Geometry check sheet. Reference: drawing and pictorial views, mm from the part's lowest x, y, z. A direction names the side the tool comes from. Round coordinates to 2 decimals unless told otherwise and drop trailing zeros. Write each loop counter-clockwise with the first axis right and the second up, starting at its lowest first coordinate (ties: lowest second). Pieces come first, ordered by that corner, then holes. Notation, with made-up numbers: M -37.5,89.5 L 1.5,89.5 A17 ccw 1.5,112.5 Z; hole C -39.75,5.25 d5. An arc over 180 degrees is marked long. Put each result on its own line as item: value. Start each with the question number.
(1) Gauge pin test, flat end, axial feed: pin 1 (3 mm diameter, centred on y = 2, z = 4, fed in from +X). Record the tip position at first contact, or that the pin passes through.
(2) Section check D-D on z = 0.55. Record the cut outline in (x, y).
(3) Tool access check on the marked faces 1 and 2. Record the directions out of +Z, -Z, +X, -X, +Y, -Y that give a thin tool (end or side, any length) a straight path to the whole face; none if there is none.
(4) Material ranges on probe 1 along Z at (x, y) = (3.35, 6) (1 decimal); probe 2 along Y at (x, z) = (3.75, 4.6); probe 3 along Z at (x, y) = (2.5, 3.5), recorded low to high.
(5) Mould release check, pull along X, two halves, no side actions. Record for the marked faces 3, 4 and 5: pulls with the +X half, pulls with the -X half, needs draft (parallel to the pull), parting line crosses it, or undercut.
(6) Section check C-C on y = 8.75. Record the cut outline in (x, z) (1 decimal).
(7) Section check B-B on x = 3.6. Record the cut outline in (y, z).
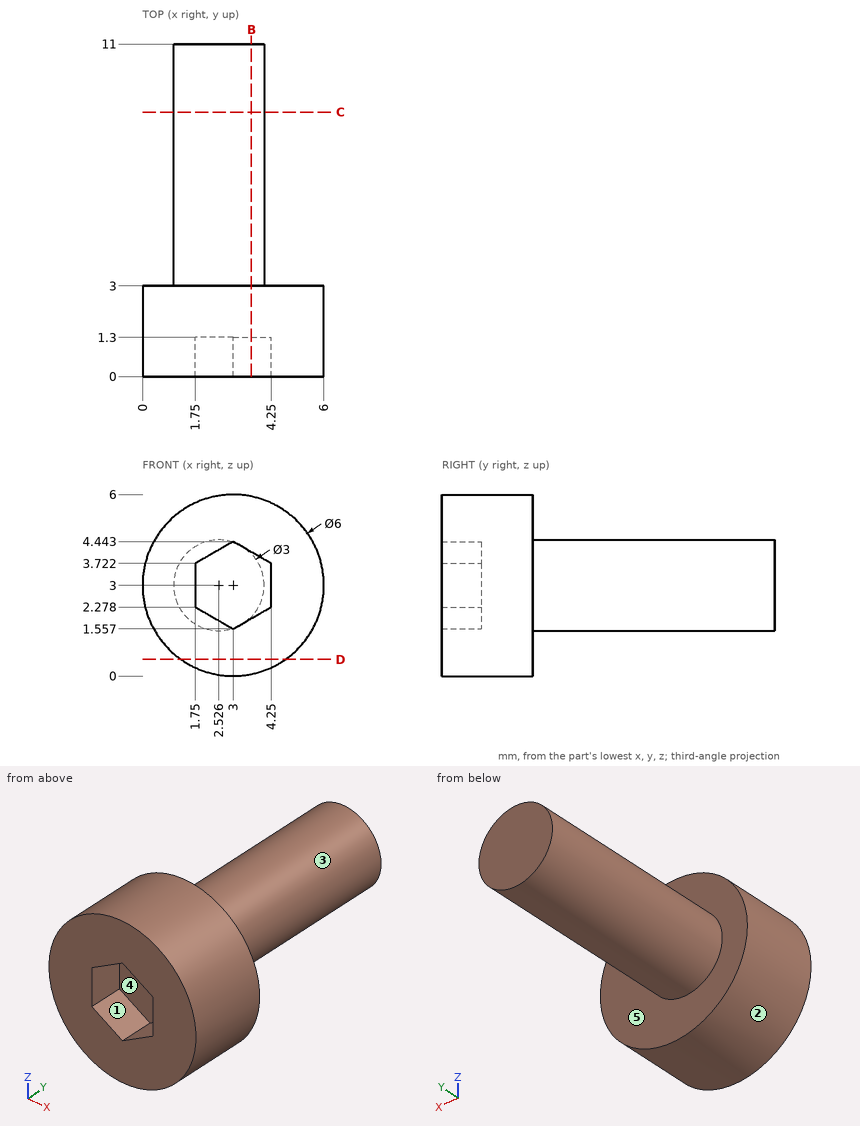
Answers follow:
1. pin 1: stops at x = 6
2. outline: M 1.27,0 L 4.73,0 L 4.73,3 L 1.27,3 Z
3. face 1: -Y
3. face 2: +Y, -Y
4. probe 1: z = 1.7 to 4.3
4. probe 2: y = 0 to 3
4. probe 3: z = 1.5 to 4.5
5. face 3: parting line crosses it
5. face 4: undercut
5. face 5: needs draft
6. outline: C 2.5,3 d3
7. outline: M 0,0.06 L 3,0.06 L 3,1.95 L 11,1.95 L 11,4.05 L 3,4.05 L 3,5.94 L 0,5.94 L 0,4.1 L 1.3,4.1 L 1.3,1.9 L 0,1.9 Z
